Input: dimensioned drawing with shaded views. Units: mm. Origin: part minimum x, y, z. A direction names the side the tool comes from. Give positions to 0.01 mm unless a question says otherwise; leave off trailing zeros. Loops run counter-clockwise (first coordinate to the right, second up) from the corner with the lowest first, then second, coordinate; pieces in that order, holes last.
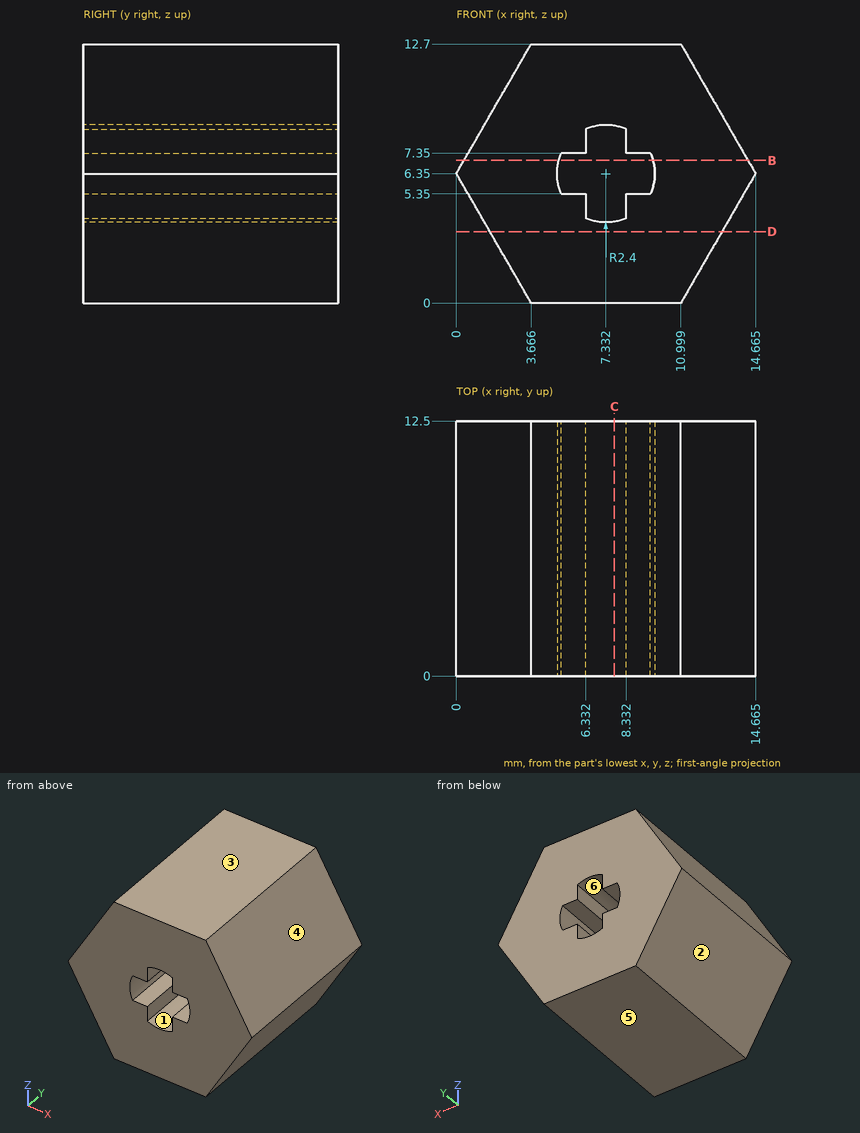
Item 1: Ray query, probe 1 along Z at (x, y) = (9, 5.75); probe 2 along X at (y, z) = (9.5, 4.25); probe 3 along Z at (x, y) = (8, 1) (1 decimal). Return the intervals inside material, ascending.
Values follow:
probe 1: z = 0 to 5.35, 7.35 to 12.7
probe 2: x = 1.21 to 6.33, 8.33 to 13.45
probe 3: z = 0 to 4, 8.7 to 12.7
Item 2: Section query B-B on z = 7. Return loops of the section in (x, y) (1 decimal), plus the area to 3 significant figures.
Values follow:
outline: (0.4, 0) - (5, 0) - (5, 12.5) - (0.4, 12.5) - close; (9.6, 0) - (14.3, 0) - (14.3, 12.5) - (9.6, 12.5) - close
area: 116 mm2
Item 3: Draft query along X for the marked faces 1, 2, 3 and 4. Return one class per face: +X half, -X half, draft (parallel to the pull), parting line (faces both ways), or undercut.
Values follow:
face 1: undercut
face 2: -X half
face 3: draft
face 4: +X half
Item 4: Pin query (flat end, axial travel): pin 1 (1.5 mm diameter, centred on y = 7.5, z = 10.5, fed in from +X); pin 2 (0.9 mm diameter, centred on y = 4.5, z = 8, fed in from +X); pin 3 (1.3 mm diameter, centred on y = 7.5, z = 8, fed in from -X). Return the tip coordinate at first contact, or that it passes through.
Values follow:
pin 1: stops at x = 12.7
pin 2: stops at x = 13.97
pin 3: stops at x = 0.58
Item 5: Section query C-C on x = 7.75. Return loops of the section in (y, z).
Values follow:
outline: (0, 0) - (12.5, 0) - (12.5, 3.99) - (0, 3.99) - close; (0, 8.71) - (12.5, 8.71) - (12.5, 12.7) - (0, 12.7) - close
Item 6: Section query D-D on z = 3.5. Return loops of the section in (x, y) (1 decimal).
Values follow:
outline: (1.6, 0) - (13, 0) - (13, 12.5) - (1.6, 12.5) - close
Item 7: Set-up query: the marked faces 5 and 6. Return all of +Z, -Z, +X, -X, +Y, -Y with unobstructed straight access to the full face (end or side cutting, diameter ignored); none if empty.
Values follow:
face 5: -Z, +X, -X, +Y, -Y
face 6: +Y, -Y
